Read the model definition and answer for the solid it produces. Units are mm, in the model's axes. A direction names the side the tool comes from. Round coordinates to 2 decimals unless told otherwise and drop trailing zeros. Write each loop counter-clockwise with the first axis right and the second up, starting at its lowest first coordinate (ties: lowest second). Pieces come first, ordered by that corner, then holes. Notation, with made-up numbers: (31.25, -4.5) - (40.25, -4.5) arc R15 ccw to (40.25, 6.5) - close; hole circle Ø4 at (23, 79). An arc over 180 degrees is marked (long way). One line per item, written item: value. Start each with the question number.
(1) For faces 1 (the face through (66.1, 0, -3)), 2 (the face through (-51.5, 14, 2)), 3 (the face through (60, -12.55, 2)), 4 (the face through (-51.5, -14, 2)), determine the directions among +Z, -Z, +X, -X, +Y, -Y from which every point of the face is accessible in a straight line to the end or side of a thin tool.
(2) A cutting plane is placed at A-A, the plane z = -2. Determine the outline of the cut face in (x, y).
(3) A cutting plane is placed at B-B, the plane x = -45.5. Determine the outline of the cut face in (y, z).
(4) The mould has two halves that part along X. Classify faces 5 (the face through (72, 0, -3.4)), 6 (the face through (-76.9, -8.7, -4.5)), 7 (the face through (72.572, -1.095, -4.534)), 8 (the face through (66, 11.7, 0.2)): +X half, -X half, draft (parallel to the pull), parting line (faces both ways), or undercut.
(5) Find the intervals of material crossed by L1, parallel to Y at x = -74.35, z = -4.2; L2, parallel to X at y = -2.5, z = -2.5; L3, parallel to X at y = 2.5, z = -1, in increasing order.
(6) Flat-ended cylindrical pins translate along their axes: pin 1 Ø3.5 at (x, y) = (-74.35, -6.14) entering from +Z; pin 2 Ø0.8 at (x, y) = (-58, 14) entering from +Z; pin 3 Ø3 at (y, z) = (-5.5, -1) entering from -X; pin 4 Ø5 at (x, z) = (43.5, 3) entering from -Y. Find the tip coordinate at first contact, or state that the pin passes through.
from build123d import *

# Parameters (mm, degrees)
F0_W          = 24
F0_H          = 12
F1_DEPTH      = 4.5
F2_W          = 134.0499658869
F2_H          = 37.3212727123
F3_DEPTH      = 1.3
F5_DEPTH      = 2.6
F6_R          = 1.8
F6_R_2        = 1.8546222436
F7_DEPTH      = 6.3
F8_W          = 131.4748737342
F8_H          = 57.6514146297
F9_DEPTH      = 5.7
F10_R         = 1.175
F11_DEPTH     = 2
F12_R         = 1.8546222436
F12_R_2       = 1.8
F13_DEPTH     = 4
F14_T1_DEPTH  = 24
F14_T3_DEPTH  = 12
F14_T9_DEPTH  = 15.5707142143
F14_T13_DEPTH = 27.5707142143
F14_T20_DEPTH = 27.5707142143
F14_T24_DEPTH = 15.5707142143
F14_T31_DEPTH = 15.5707142143
F14_T35_DEPTH = 27.5707142143
F14_T42_DEPTH = 27.5707142143
F14_T46_DEPTH = 15.5707142143


# Not quite as in the source:
# - a fillet or chamfer that OpenCascade refuses, or shapes differently, is made with other operations: its cross-section is extruded or revolved along the edge and cut away or added


with BuildPart() as f1:
    # F0 (on Top) → F1 (new body)
    with BuildSketch(Plane.XY):
        Polygon((-51.5, 15), (-66, 15), (-66, 10), (-63.8, 10), (-63.8, -10), (-66, -10), (-66, -15), (-51.5, -15), (-51.5, -12.55), (52.5, -12.55), (52.5, -15), (66, -15), (66, 15), (53.5, 15), (53.5, 12.55), (-51.5, 12.55), align=None)
        Rectangle(F0_W, F0_H, mode=Mode.SUBTRACT)
    extrude(amount=F1_DEPTH)

    # F2 (on face) → F3 (cut)
    with BuildSketch(Plane.XY.offset(4.5)):
        with Locations((3.2249829435, -1.1242744513)):
            Rectangle(F2_W, F2_H)
    extrude(amount=-F3_DEPTH, mode=Mode.SUBTRACT)

    # F4 (on face) → F5 (cut)
    with BuildSketch(Plane.XY.offset(3.2)):
        Polygon((-63.8, 12.5), (-63.8, -12.55), (-51.5, -12.55), (-51.5, -30.0471726805), (53.5, -30.0471726805), (53.5, -12.55), (68.7586962298, -12.55), (68.7586962298, 12.5), (53.5, 12.55), (53.5, 21.0785120726), (-51.5, 21.0785120726), (-51.5, 12.55), align=None)
    extrude(amount=-F5_DEPTH, mode=Mode.SUBTRACT)

    # F6 (on face) → F7 (join)
    with BuildSketch(Plane.XY.offset(0.6)):
        with BuildLine():
            Line((66, 3.5), (66, -3.5))
            Line((66, -3.5), (74.1, -3.5))
            ThreePointArc((74.1, -3.5), (76.5748737342, -2.4748737342), (77.6, 0))
            ThreePointArc((77.6, 0), (76.5748737342, 2.4748737342), (74.1, 3.5))
            Line((74.1, 3.5), (66, 3.5))
        make_face()
        with Locations((74, 0)):
            Circle(F6_R, mode=Mode.SUBTRACT)
        with BuildLine():
            Line((-74.4, -9.75), (-63.8, -9.75))
            Line((-63.8, -9.75), (-63.8, -2.25))
            Line((-63.8, -2.25), (-74.4, -2.25))
            ThreePointArc((-74.4, -2.25), (-76.8748737342, -3.2751262658), (-77.9, -5.75))
            Line((-77.9, -5.75), (-77.9, -6.25))
            ThreePointArc((-77.9, -6.25), (-76.8748737342, -8.7248737342), (-74.4, -9.75))
        make_face()
        with Locations((-74.35, -6.136629995)):
            Circle(F6_R_2, mode=Mode.SUBTRACT)
    extrude(amount=-F7_DEPTH)

    # F8 (on face) → F9 (cut, through all)
    with BuildSketch(Plane(origin=(0, 0, -5.7), x_dir=(1, 0, 0), z_dir=(0, 0, -1))):
        with Locations((0.3625631329, -2.5597326458)):
            Rectangle(F8_W, F8_H)
    extrude(amount=-F9_DEPTH, mode=Mode.SUBTRACT)

    # F10 (on face) → F11 (cut)
    with BuildSketch(Plane(origin=(0, 0, 0), x_dir=(1, 0, 0), z_dir=(0, 0, -1))):
        with Locations((55.875, -5.075)):
            Circle(F10_R)
    extrude(amount=-F11_DEPTH, mode=Mode.SUBTRACT)

    # F12 (on face) → F13 (cut)
    with BuildSketch(Plane.XY.offset(0.6)):
        with BuildLine():
            Line((-69.0248737342, -9.75), (-69.0248737342, -2.25))
            Line((-69.0248737342, -2.25), (-74.4, -2.25))
            ThreePointArc((-74.4, -2.25), (-76.8748737342, -3.2751262658), (-77.9, -5.75))
            Line((-77.9, -5.75), (-77.9, -6.25))
            ThreePointArc((-77.9, -6.25), (-76.8748737342, -8.7248737342), (-74.4, -9.75))
            Line((-74.4, -9.75), (-69.0248737342, -9.75))
        make_face()
        with Locations((-74.35, -6.136629995)):
            Circle(F12_R, mode=Mode.SUBTRACT)
        with BuildLine():
            Line((74.1, 3.5), (69.75, 3.5))
            Line((69.75, 3.5), (69.75, -3.5))
            Line((69.75, -3.5), (74.1, -3.5))
            ThreePointArc((74.1, -3.5), (77.6, 0), (74.1, 3.5))
        make_face()
        with Locations((74, 0)):
            Circle(F12_R_2, mode=Mode.SUBTRACT)
    extrude(amount=-F13_DEPTH, mode=Mode.SUBTRACT)

    # F14: fillet of radius 2 on 4 edges, made by hand

    # F14_s2 → F14_t1 (cut)
    with BuildSketch(Plane.YZ.offset(-12)):
        with BuildLine():
            ThreePointArc((6, 0), (6.6536890165, 0.4439088915), (7.4282856857, 0.6))
            Line((7.4282856857, 0.6), (6, 0.6))
            Line((6, 0.6), (6, 0))
        make_face()
        with BuildLine():
            ThreePointArc((-6, 0), (-6.6536890165, 0.4439088915), (-7.4282856857, 0.6))
            Line((-7.4282856857, 0.6), (-6, 0.6))
            Line((-6, 0.6), (-6, 0))
        make_face()
    extrude(amount=F14_T1_DEPTH, mode=Mode.SUBTRACT)

    # F14_s4 → F14_t3 (cut)
    with BuildSketch(Plane.XZ.offset(-6)):
        with BuildLine():
            ThreePointArc((-12, 0), (-12.6536890165, 0.4439088915), (-13.4282856857, 0.6))
            Line((-13.4282856857, 0.6), (-12, 0.6))
            Line((-12, 0.6), (-12, 0))
        make_face()
        with BuildLine():
            ThreePointArc((12, 0), (12.6536890165, 0.4439088915), (13.4282856857, 0.6))
            Line((13.4282856857, 0.6), (12, 0.6))
            Line((12, 0.6), (12, 0))
        make_face()
    extrude(amount=F14_T3_DEPTH, mode=Mode.SUBTRACT)


with BuildPart() as f14_tool7:
    # F14_s8 → F14_t9 (new body)
    with BuildSketch(Plane.XZ.offset(6)):
        with BuildLine():
            ThreePointArc((-12, 0), (-12.6536890165, 0.4439088915), (-13.4282856857, 0.6))
            Line((-13.4282856857, 0.6), (-12, 0.6))
            Line((-12, 0.6), (-12, 0))
        make_face()
    extrude(amount=-F14_T9_DEPTH)

    split(bisect_by=Plane.XZ.offset(-6), keep=Keep.BOTTOM)


with BuildPart() as f14_tool11:
    # F14_s12 → F14_t13 (new body)
    with BuildSketch(Plane.YZ.offset(-15.5707142143)):
        with BuildLine():
            ThreePointArc((6, 0), (6.6536890165, 0.4439088915), (7.4282856857, 0.6))
            Line((7.4282856857, 0.6), (6, 0.6))
            Line((6, 0.6), (6, 0))
        make_face()
    extrude(amount=F14_T13_DEPTH)

    split(bisect_by=Plane.YZ.offset(-12), keep=Keep.BOTTOM)


with BuildPart() as f14_tool7_1:
    add(f14_tool7.part)

    # F14_t15: intersect F14_tool11
    add(f14_tool11.part, mode=Mode.INTERSECT)


with BuildPart() as f1_1:
    add(f1.part)

    # F14_t5: cut F14_tool7
    add(f14_tool7_1.part, mode=Mode.SUBTRACT)


with BuildPart() as f14_tool18:
    # F14_s19 → F14_t20 (new body)
    with BuildSketch(Plane.YZ.offset(-12)):
        with BuildLine():
            ThreePointArc((6, 0), (6.6536890165, 0.4439088915), (7.4282856857, 0.6))
            Line((7.4282856857, 0.6), (6, 0.6))
            Line((6, 0.6), (6, 0))
        make_face()
    extrude(amount=F14_T20_DEPTH)

    split(bisect_by=Plane.YZ.offset(12), keep=Keep.TOP)


with BuildPart() as f14_tool22:
    # F14_s23 → F14_t24 (new body)
    with BuildSketch(Plane.XZ.offset(-9.5707142143)):
        with BuildLine():
            ThreePointArc((12, 0), (12.6536890165, 0.4439088915), (13.4282856857, 0.6))
            Line((13.4282856857, 0.6), (12, 0.6))
            Line((12, 0.6), (12, 0))
        make_face()
    extrude(amount=F14_T24_DEPTH)

    split(bisect_by=Plane.XZ.offset(-6), keep=Keep.BOTTOM)


with BuildPart() as f14_tool18_1:
    add(f14_tool18.part)

    # F14_t26: intersect F14_tool22
    add(f14_tool22.part, mode=Mode.INTERSECT)


with BuildPart() as f1_2:
    add(f1_1.part)

    # F14_t16: cut F14_tool18
    add(f14_tool18_1.part, mode=Mode.SUBTRACT)


with BuildPart() as f14_tool29:
    # F14_s30 → F14_t31 (new body)
    with BuildSketch(Plane.XZ.offset(9.5707142143)):
        with BuildLine():
            ThreePointArc((-12, 0), (-12.6536890165, 0.4439088915), (-13.4282856857, 0.6))
            Line((-13.4282856857, 0.6), (-12, 0.6))
            Line((-12, 0.6), (-12, 0))
        make_face()
    extrude(amount=-F14_T31_DEPTH)

    split(bisect_by=Plane.XZ.offset(6), keep=Keep.TOP)


with BuildPart() as f14_tool33:
    # F14_s34 → F14_t35 (new body)
    with BuildSketch(Plane.YZ.offset(12)):
        with BuildLine():
            ThreePointArc((-6, 0), (-6.6536890165, 0.4439088915), (-7.4282856857, 0.6))
            Line((-7.4282856857, 0.6), (-6, 0.6))
            Line((-6, 0.6), (-6, 0))
        make_face()
    extrude(amount=-F14_T35_DEPTH)

    split(bisect_by=Plane.YZ.offset(-12), keep=Keep.BOTTOM)


with BuildPart() as f14_tool29_1:
    add(f14_tool29.part)

    # F14_t37: intersect F14_tool33
    add(f14_tool33.part, mode=Mode.INTERSECT)


with BuildPart() as f1_3:
    add(f1_2.part)

    # F14_t27: cut F14_tool29
    add(f14_tool29_1.part, mode=Mode.SUBTRACT)


with BuildPart() as f14_tool40:
    # F14_s41 → F14_t42 (new body)
    with BuildSketch(Plane.YZ.offset(15.5707142143)):
        with BuildLine():
            ThreePointArc((-6, 0), (-6.6536890165, 0.4439088915), (-7.4282856857, 0.6))
            Line((-7.4282856857, 0.6), (-6, 0.6))
            Line((-6, 0.6), (-6, 0))
        make_face()
    extrude(amount=-F14_T42_DEPTH)

    split(bisect_by=Plane.YZ.offset(12), keep=Keep.TOP)


with BuildPart() as f14_tool44:
    # F14_s45 → F14_t46 (new body)
    with BuildSketch(Plane.XZ.offset(-6)):
        with BuildLine():
            ThreePointArc((12, 0), (12.6536890165, 0.4439088915), (13.4282856857, 0.6))
            Line((13.4282856857, 0.6), (12, 0.6))
            Line((12, 0.6), (12, 0))
        make_face()
    extrude(amount=F14_T46_DEPTH)

    split(bisect_by=Plane.XZ.offset(6), keep=Keep.TOP)


with BuildPart() as f14_tool40_1:
    add(f14_tool40.part)

    # F14_t48: intersect F14_tool44
    add(f14_tool44.part, mode=Mode.INTERSECT)


with BuildPart() as f1_4:
    add(f1_3.part)

    # F14_t38: cut F14_tool40
    add(f14_tool40_1.part, mode=Mode.SUBTRACT)


solid = f1_4.part
Here are the results:
1. face 1: -Z, +Y, -Y
1. face 2: +Z, -Z, +Y
1. face 3: +Z, +X
1. face 4: +Z, -Z, -Y
2. outline: (-69.02, -9.75) - (-65.37, -9.75) - (-65.37, -2.25) - (-69.02, -2.25) - close; (66.1, -3.5) - (69.75, -3.5) - (69.75, 3.5) - (66.1, 3.5) - close
3. outline: (-12.55, 0) - (12.55, 0) - (12.55, 0.6) - (-12.55, 0.6) - close
4. face 5: draft
4. face 6: -X half
4. face 7: undercut
4. face 8: +X half
5. L1: -9.75 to -7.99, -4.28 to -2.25
5. L2: -69.02 to -65.37, 66.1 to 69.75
5. L3: 66.1 to 69.75
6. pin 1: through
6. pin 2: z = 3.2
6. pin 3: x = -69.02
6. pin 4: y = -12.55
